from build123d import *

# Parameters (mm, degrees)
F0_W     = 100
F0_H     = 91
F0_W_2   = 60
F0_H_2   = 2.0199990959
F0_W_3   = 20
F0_H_3   = 5
F0_H_4   = 0.9000000043
F1_DEPTH = 2.5
F2_DEPTH = 8
F3_DEPTH = 8
F4_DEPTH = 25


with BuildPart() as f1:
    # F0 (on Top) → F1 (new body)
    with BuildSketch(Plane.XY):
        with Locations((41.1687159911, -7.0227757916)):
            Rectangle(F0_W, F0_H)
        Polygon((-1.7512831092, 31.3972233087), (11.1687159911, 31.3972233087), (71.1687159911, 31.3972233087), (84.0887150913, 31.3972233087), (84.0887150913, -45.4427748919), (71.1687159911, -45.4427748919), (11.1687159911, -45.4427748919), (-1.7512831092, -45.4427748919), align=None, mode=Mode.SUBTRACT)
        with BuildLine():
            Line((71.1687159911, 28.4772242084), (11.1687159911, 28.4772242084))
            Line((11.1687159911, 28.4772242084), (11.1687159911, 28.1993557262))
            ThreePointArc((11.1687159911, 28.1993557262), (12.5467403812, 27.1370434757), (13.0687159911, 25.4772242084))
            ThreePointArc((13.0687159911, 25.4772242084), (12.5467403812, 23.8174049411), (11.1687159911, 22.7550926907))
            Line((11.1687159911, 22.7550926907), (11.1687159911, -42.5227757916))
            Line((11.1687159911, -42.5227757916), (31.1687159911, -42.5227757916))
            Line((31.1687159911, -42.5227757916), (31.1687159911, -37.5227757916))
            Line((31.1687159911, -37.5227757916), (51.1687159911, -37.5227757916))
            Line((51.1687159911, -37.5227757916), (51.1687159911, -42.5227757916))
            Line((51.1687159911, -42.5227757916), (71.1687159911, -42.5227757916))
            Line((71.1687159911, -42.5227757916), (71.1687159911, 22.7550926907))
            ThreePointArc((71.1687159911, 22.7550926907), (69.2687159911, 25.4772242084), (71.1687159911, 28.1993557262))
            Line((71.1687159911, 28.1993557262), (71.1687159911, 28.4772242084))
        make_face()
        with BuildLine():
            Line((11.1687159911, 28.4772242084), (1.1687159911, 28.4772242084))
            Line((1.1687159911, 28.4772242084), (1.1687159911, -42.5227757916))
            Line((1.1687159911, -42.5227757916), (11.1687159911, -42.5227757916))
            Line((11.1687159911, -42.5227757916), (11.1687159911, 22.7550926907))
            ThreePointArc((11.1687159911, 22.7550926907), (7.2687159911, 25.4772242084), (11.1687159911, 28.1993557262))
            Line((11.1687159911, 28.1993557262), (11.1687159911, 28.4772242084))
        make_face()
        with BuildLine():
            Line((81.1687159911, 28.4772242084), (71.1687159911, 28.4772242084))
            Line((71.1687159911, 28.4772242084), (71.1687159911, 28.1993557262))
            ThreePointArc((71.1687159911, 28.1993557262), (73.8285352583, 27.8552485985), (75.0687159911, 25.4772242084))
            ThreePointArc((75.0687159911, 25.4772242084), (73.8285352583, 23.0991998183), (71.1687159911, 22.7550926907))
            Line((71.1687159911, 22.7550926907), (71.1687159911, -42.5227757916))
            Line((71.1687159911, -42.5227757916), (81.1687159911, -42.5227757916))
            Line((81.1687159911, -42.5227757916), (81.1687159911, 28.4772242084))
        make_face()
        Polygon((0.2687159867, 29.3772242127), (11.1687159911, 29.3772242127), (11.1687159911, 31.3972233087), (-1.7512831092, 31.3972233087), (-1.7512831092, -45.4427748919), (11.1687159911, -45.4427748919), (11.1687159911, -43.4227757959), (0.2687159867, -43.4227757959), align=None)
        Polygon((71.1687159911, 31.3972233087), (71.1687159911, 29.3772242127), (82.0687159954, 29.3772242127), (82.0687159954, -43.4227757959), (71.1687159911, -43.4227757959), (71.1687159911, -45.4427748919), (84.0887150913, -45.4427748919), (84.0887150913, 31.3972233087), align=None)
        with Locations((41.1687159911, 30.3872237607)):
            Rectangle(F0_W_2, F0_H_2)
        with Locations((41.1687159911, -44.4327753439)):
            Rectangle(F0_W_2, F0_H_2)
        with Locations((41.1687159911, -40.0227757916)):
            Rectangle(F0_W_3, F0_H_3)
        Polygon((1.1687159911, -42.5227757916), (1.1687159911, 28.4772242084), (11.1687159911, 28.4772242084), (11.1687159911, 29.3772242127), (0.2687159867, 29.3772242127), (0.2687159867, -43.4227757959), (11.1687159911, -43.4227757959), (11.1687159911, -42.5227757916), align=None)
        Polygon((71.1687159911, 29.3772242127), (71.1687159911, 28.4772242084), (81.1687159911, 28.4772242084), (81.1687159911, -42.5227757916), (71.1687159911, -42.5227757916), (71.1687159911, -43.4227757959), (82.0687159954, -43.4227757959), (82.0687159954, 29.3772242127), align=None)
        with Locations((41.1687159911, 28.9272242106)):
            Rectangle(F0_W_2, F0_H_4)
        Polygon((31.1687159911, -42.5227757916), (11.1687159911, -42.5227757916), (11.1687159911, -43.4227757959), (71.1687159911, -43.4227757959), (71.1687159911, -42.5227757916), (51.1687159911, -42.5227757916), align=None)
        with BuildLine():
            Line((11.1687159911, 26.3078865947), (11.1687159911, 28.1993557262))
            ThreePointArc((11.1687159911, 28.1993557262), (7.2687159911, 25.4772242084), (11.1687159911, 22.7550926907))
            Line((11.1687159911, 22.7550926907), (11.1687159911, 24.6465618221))
            ThreePointArc((11.1687159911, 24.6465618221), (8.8687159911, 25.4772242084), (11.1687159911, 26.3078865947))
        make_face()
        with BuildLine():
            ThreePointArc((75.0687159911, 25.4772242084), (73.8285352583, 27.8552485985), (71.1687159911, 28.1993557262))
            Line((71.1687159911, 28.1993557262), (71.1687159911, 26.3078865947))
            ThreePointArc((71.1687159911, 26.3078865947), (72.6103040344, 26.6999261345), (73.4687159911, 25.4772242084))
            ThreePointArc((73.4687159911, 25.4772242084), (72.6103040344, 24.2545222824), (71.1687159911, 24.6465618221))
            Line((71.1687159911, 24.6465618221), (71.1687159911, 22.7550926907))
            ThreePointArc((71.1687159911, 22.7550926907), (73.8285352583, 23.0991998183), (75.0687159911, 25.4772242084))
        make_face()
        with BuildLine():
            ThreePointArc((13.0687159911, 25.4772242084), (12.5467403812, 27.1370434757), (11.1687159911, 28.1993557262))
            Line((11.1687159911, 28.1993557262), (11.1687159911, 26.3078865947))
            ThreePointArc((11.1687159911, 26.3078865947), (11.3914179171, 25.9188122517), (11.4687159911, 25.4772242084))
            ThreePointArc((11.4687159911, 25.4772242084), (11.3914179171, 25.0356361651), (11.1687159911, 24.6465618221))
            Line((11.1687159911, 24.6465618221), (11.1687159911, 22.7550926907))
            ThreePointArc((11.1687159911, 22.7550926907), (12.5467403812, 23.8174049411), (13.0687159911, 25.4772242084))
        make_face()
        with BuildLine():
            Line((71.1687159911, 26.3078865947), (71.1687159911, 28.1993557262))
            ThreePointArc((71.1687159911, 28.1993557262), (69.2687159911, 25.4772242084), (71.1687159911, 22.7550926907))
            Line((71.1687159911, 22.7550926907), (71.1687159911, 24.6465618221))
            ThreePointArc((71.1687159911, 24.6465618221), (70.8687159911, 25.4772242084), (71.1687159911, 26.3078865947))
        make_face()
    extrude(amount=-F1_DEPTH)

    # F0 (on Top) → F2 (join)
    with BuildSketch(Plane.XY):
        with Locations((41.1687159911, -40.0227757916)):
            Rectangle(F0_W_3, F0_H_3)
        with BuildLine():
            Line((11.1687159911, 26.3078865947), (11.1687159911, 28.1993557262))
            ThreePointArc((11.1687159911, 28.1993557262), (7.2687159911, 25.4772242084), (11.1687159911, 22.7550926907))
            Line((11.1687159911, 22.7550926907), (11.1687159911, 24.6465618221))
            ThreePointArc((11.1687159911, 24.6465618221), (8.8687159911, 25.4772242084), (11.1687159911, 26.3078865947))
        make_face()
        with BuildLine():
            ThreePointArc((13.0687159911, 25.4772242084), (12.5467403812, 27.1370434757), (11.1687159911, 28.1993557262))
            Line((11.1687159911, 28.1993557262), (11.1687159911, 26.3078865947))
            ThreePointArc((11.1687159911, 26.3078865947), (11.3914179171, 25.9188122517), (11.4687159911, 25.4772242084))
            ThreePointArc((11.4687159911, 25.4772242084), (11.3914179171, 25.0356361651), (11.1687159911, 24.6465618221))
            Line((11.1687159911, 24.6465618221), (11.1687159911, 22.7550926907))
            ThreePointArc((11.1687159911, 22.7550926907), (12.5467403812, 23.8174049411), (13.0687159911, 25.4772242084))
        make_face()
        with BuildLine():
            Line((71.1687159911, 26.3078865947), (71.1687159911, 28.1993557262))
            ThreePointArc((71.1687159911, 28.1993557262), (69.2687159911, 25.4772242084), (71.1687159911, 22.7550926907))
            Line((71.1687159911, 22.7550926907), (71.1687159911, 24.6465618221))
            ThreePointArc((71.1687159911, 24.6465618221), (70.8687159911, 25.4772242084), (71.1687159911, 26.3078865947))
        make_face()
        with BuildLine():
            ThreePointArc((75.0687159911, 25.4772242084), (73.8285352583, 27.8552485985), (71.1687159911, 28.1993557262))
            Line((71.1687159911, 28.1993557262), (71.1687159911, 26.3078865947))
            ThreePointArc((71.1687159911, 26.3078865947), (72.6103040344, 26.6999261345), (73.4687159911, 25.4772242084))
            ThreePointArc((73.4687159911, 25.4772242084), (72.6103040344, 24.2545222824), (71.1687159911, 24.6465618221))
            Line((71.1687159911, 24.6465618221), (71.1687159911, 22.7550926907))
            ThreePointArc((71.1687159911, 22.7550926907), (73.8285352583, 23.0991998183), (75.0687159911, 25.4772242084))
        make_face()
    extrude(amount=F2_DEPTH)

    # F0 (on Top) → F3 (join)
    with BuildSketch(Plane.XY):
        Polygon((0.2687159867, 29.3772242127), (11.1687159911, 29.3772242127), (11.1687159911, 31.3972233087), (-1.7512831092, 31.3972233087), (-1.7512831092, -45.4427748919), (11.1687159911, -45.4427748919), (11.1687159911, -43.4227757959), (0.2687159867, -43.4227757959), align=None)
        Polygon((71.1687159911, 31.3972233087), (71.1687159911, 29.3772242127), (82.0687159954, 29.3772242127), (82.0687159954, -43.4227757959), (71.1687159911, -43.4227757959), (71.1687159911, -45.4427748919), (84.0887150913, -45.4427748919), (84.0887150913, 31.3972233087), align=None)
    extrude(amount=F3_DEPTH)

    # F0 (on Top) → F4 (join)
    with BuildSketch(Plane.XY):
        with Locations((41.1687159911, -44.4327753439)):
            Rectangle(F0_W_2, F0_H_2)
    extrude(amount=F4_DEPTH)


solid = f1.part
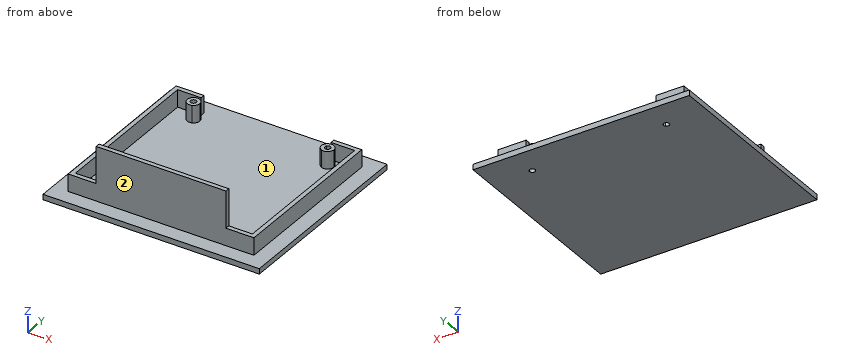
Can you work these out from the model? Positions are in its coordinate system, mm. Face numbers are marked on the shaded views. Round coordinates to 2 decimals unless told otherwise and drop trailing zeros. Order: outer loops, then holes, each group sorted by start corner. A loop starts at its lowest first (then second) coordinate and runs counter-clockwise, first axis right, second up. Notation, with made-up numbers: (81.5, 25.25) - (88.5, 25.25) arc R36 cw to (88.5, 61.25) - close; hole circle Ø11 at (62, 88). An arc over 180 degrees is marked (long way). Answer in a Markdown table with one row per item.
(1) Suppose I cut it at D-D, the plane y = -21. Please give me the cut outline in (x, z), plus the area to 3 significant figures.
From the geometry:
| item | result |
|---|---|
| outline | (-8.83, -2.5) - (91.17, -2.5) - (91.17, 0) - (84.09, 0) - (84.09, 8) - (82.07, 8) - (82.07, 0) - (0.27, 0) - (0.27, 8) - (-1.75, 8) - (-1.75, 0) - (-8.83, 0) - close |
| area | 282 mm2 |
(2) Suppose I cut it at C-C, the plane z = 16.25. Please give me the cut outline in (x, y), plus the area to 3 significant figures.
From the geometry:
| item | result |
|---|---|
| outline | (11.17, -45.44) - (71.17, -45.44) - (71.17, -43.42) - (11.17, -43.42) - close |
| area | 121 mm2 |
(3) Please list where these lines run through material, in increasing order: L1, parallel to X at y = -40, z = 4; L2, parallel to Y at x = 43, z = 4; L3, parallel to X at y = -11.5, z = 4.25. Write a range as from..to.
From the geometry:
| item | result |
|---|---|
| L1 | x = -1.75..0.27, 31.17..51.17, 82.07..84.09 |
| L2 | y = -45.44..-43.42, -42.52..-37.52 |
| L3 | x = -1.75..0.27, 82.07..84.09 |
(4) If we mould it in two halves opening along X, with no side actions, what happens to the marked faces 1 and 2? For each: released by +X, released by -X, zero draft, split by the parting line, or undercut.
From the geometry:
| item | result |
|---|---|
| face 1 | undercut |
| face 2 | zero draft |
(5) Suppose I cut it at B-B, the plane x = 4.5. Please give me the cut outline in (y, z).
From the geometry:
| item | result |
|---|---|
| outline | (-52.52, -2.5) - (38.48, -2.5) - (38.48, 0) - (31.4, 0) - (31.4, 8) - (29.38, 8) - (29.38, 0) - (-43.42, 0) - (-43.42, 8) - (-45.44, 8) - (-45.44, 0) - (-52.52, 0) - close |
(6) Suppose I cut it at A-A, the plane y = -40. Please give me the cut outline in (x, z).
From the geometry:
| item | result |
|---|---|
| outline | (-8.83, -2.5) - (91.17, -2.5) - (91.17, 0) - (84.09, 0) - (84.09, 8) - (82.07, 8) - (82.07, 0) - (51.17, 0) - (51.17, 8) - (31.17, 8) - (31.17, 0) - (0.27, 0) - (0.27, 8) - (-1.75, 8) - (-1.75, 0) - (-8.83, 0) - close |
(7) For P1, Ø9, axis at y = -15, z = 6, coming from the -X side; P2, Ø1.5, axis at x = 26.5, z = 7.5, coming from the -Y side; P3, Ø3, axis at x = 59.5, y = 0, coming from the +Z side, each with a flat end and sliding along its axis, tell me the tip position at first contact or that it passes through.
From the geometry:
| item | result |
|---|---|
| P1 | stops at x = -1.75 |
| P2 | stops at y = -45.44 |
| P3 | stops at z = 0 |
